Check sheet for the modelled part. Datum: model origin and axes. Units: mm. A direction names the side the tool comes from. Coordinates: 2 decimals unless noted, no trailing zeros. Order: outer loops, then holes, each group sorted by start corner. A loop starts at its lowest first (then second) coordinate and runs counter-clockwise, first axis right, second up. Notation, with made-up numbers: (63.25, -19.5) -> (99.25, -19.5) arc R19 cw to (99.25, -13.5) -> close; hole circle Ø3 at (75.5, -24). An arc over 180 degrees is marked (long way). Put each result on its own line as item: value. Start each with the question number.
```python
from build123d import *

# Parameters (mm, degrees)
BOSS_EXTRUDE1_DEPTH = 15
SKETCH2_R           = 9
CUT_EXTRUDE1_DEPTH  = 66.5
CUT_EXTRUDE2_START  = -58
SKETCH4_R           = 11
CUT_EXTRUDE2_DEPTH  = 8
CHAMFER1_SIZE       = 17
SKETCH5_R           = 2
CUT_EXTRUDE3_DEPTH  = 105.002294435
FILLET1_R           = 10


with BuildPart() as part:
    # Sketch1 → Boss-Extrude1 (new body)
    with BuildSketch(Plane(origin=(0, 0, 0), x_dir=(1, 0, 0), z_dir=(0, 1, 0))):
        Polygon((-45, 25), (-68, 25), (-68, -77.249448203), (68, -77.249448203), (68, 25), (45, 25), (45, -45), (-45, -45), align=None)
    extrude(amount=-BOSS_EXTRUDE1_DEPTH)

    # Sketch2 → Cut-Extrude1 (cut)
    with BuildSketch(Plane(origin=(0, 0, 0), x_dir=(0, 0, -1), z_dir=(1, 0, 0))):
        Circle(SKETCH2_R)
    cut_extrude1 = extrude(amount=-CUT_EXTRUDE1_DEPTH, mode=Mode.SUBTRACT)

    # Sketch4 → Cut-Extrude2 (cut)
    with BuildSketch(Plane(origin=(0, 0, 0), x_dir=(0, 0, -1), z_dir=(1, 0, 0)).offset(CUT_EXTRUDE2_START)):
        Circle(SKETCH4_R)
    cut_extrude2 = extrude(amount=-CUT_EXTRUDE2_DEPTH, mode=Mode.SUBTRACT)

    # Chamfer1
    chamfer1_edges = [part.edges().sort_by_distance(p)[0] for p in [
        (-45, -7.5, 45),
        (45, -7.5, 45),
    ]]
    chamfer(chamfer1_edges, length=CHAMFER1_SIZE)

    # Sketch5 → Cut-Extrude3 (cut, through all)
    with BuildSketch(Plane(origin=(0, 0, 0), x_dir=(1, 0, 0), z_dir=(0, 1, 0))):
        with Locations(Location((-56.5, 19, 0), (0, 0, 270))):
            Circle(SKETCH5_R)
    cut_extrude3 = extrude(amount=-CUT_EXTRUDE3_DEPTH, mode=Mode.SUBTRACT)

    # Fillet1
    fillet1_edges = [part.edges().sort_by_distance(p)[0] for p in [
        (45, -7.5, -25),
        (68, -7.5, -25),
        (-68, -7.5, -25),
        (-45, -7.5, -25),
    ]]
    fillet(fillet1_edges, radius=FILLET1_R)

    # Mirror2: Cut-Extrude1, Cut-Extrude2, Cut-Extrude3 across plane
    add(cut_extrude1.mirror(Plane(origin=(0, 0, 0), x_dir=(0, 0, 1), z_dir=(1, 0, 0))), mode=Mode.SUBTRACT)
    add(cut_extrude2.mirror(Plane(origin=(0, 0, 0), x_dir=(0, 0, 1), z_dir=(1, 0, 0))), mode=Mode.SUBTRACT)
    add(cut_extrude3.mirror(Plane(origin=(0, 0, 0), x_dir=(0, 0, 1), z_dir=(1, 0, 0))), mode=Mode.SUBTRACT)


solid = part.part
```
1) Sectioned sample at B-B (x = 56.5). Record the boundary of the cut face in (y, z), plus the area to 3 significant figures.
2) Scan lines: line 1 along X through (y, z) = (-8, 6); line 2 along X through (y, z) = (-5.25, -19); line 3 along Z through (x, y) = (56.5, -3.5). Record each from-to range of solid material in increasing order. Write a range as [from, to].
3) Sectioned sample at A-A (z = 0). Record the boundary of the cut face in (x, y).
4) Mould release check, pull along Z, two halves, no side actions. Record for faces 4 (the flat face through (45, -9, 6)), 5 (the cylindrical face through (-47.85, -7.6, -21.99)), 6 (the cylindrical face through (54.517, -7.395, -19.26)): +Z half, -Z half, draft (parallel to the pull), parting line (faces both ways), or undercut.
5) Sectioned sample at C-C (z = -19). Record the boundary of the cut face in (x, y), plus the area to 3 significant figures.
6) Access from +Z, -Z, +X, -X, +Y, -Y to the whole of each face (thin tool, end or side, straight path). Record for faces 1 (the flat face through (-1, -15, 48)), 2 (the flat face through (0, -7, 45)), 3 (the flat face through (-66.5, -3, 0)).
7) Sectioned sample at D-D (z = 14). Record the boundary of the cut face in (x, y).
8) Gauge pin test, flat end, axial feed: pin 1 (1 mm diameter, centred on x = -12.5, y = -1.5, fed in from -Z). Record the tip position at first contact, or that the pin passes through.
Entries:
1. outline: (-15, -25) -> (0, -25) -> (0, -21) -> (-15, -21) -> close; (-15, -17) -> (0, -17) -> (0, -9) arc R9 cw to (0, 9) -> (0, 77.25) -> (-15, 77.25) -> close
1. area: 1,350 mm2
2. line 1: x = [-68, -66], [-58, -45], [45, 58], [66, 68]
2. line 2: x = [-67.17, -58.5], [-54.5, -45.83], [45.83, 54.5], [58.5, 67.17]
2. line 3: z = [-25, -21], [-17, -8.29], [8.29, 77.25]
3. outline: (-68, -15) -> (-45, -15) -> (-45, -9) -> (-58, -9) -> (-58, -11) -> (-66, -11) -> (-66, -9) -> (-66.5, -9) -> (-66.5, 0) -> (-68, 0) -> close; (45, -15) -> (68, -15) -> (68, 0) -> (66.5, 0) -> (66.5, -9) -> (66, -9) -> (66, -11) -> (58, -11) -> (58, -9) -> (45, -9) -> close
4. face 4: draft
4. face 5: -Z half
4. face 6: undercut
5. outline: (-67.17, -15) -> (-58.5, -15) -> (-58.5, 0) -> (-67.17, 0) -> close; (-54.5, -15) -> (-45.83, -15) -> (-45.83, 0) -> (-54.5, 0) -> close; (45.83, -15) -> (54.5, -15) -> (54.5, 0) -> (45.83, 0) -> close; (58.5, -15) -> (67.17, -15) -> (67.17, 0) -> (58.5, 0) -> close
5. area: 520 mm2
6. face 1: +Z, -Z, +X, -X, -Y
6. face 2: -Z, +Y, -Y
6. face 3: +Y
7. outline: (-68, -15) -> (-45, -15) -> (-45, 0) -> (-68, 0) -> close; (45, -15) -> (68, -15) -> (68, 0) -> (45, 0) -> close
8. pin 1: stops at z = 45
